The listing builds one solid part. Answer for the finished solid, in the listing's coordinates (mm). A direction names the side the tool comes from. Round coordinates to 2 decimals unless told otherwise and drop trailing zeros. Loops run counter-clockwise (first coordinate to the right, second up) from the corner with the lowest first, then second, coordinate; pieces in that order, holes last. Notation, with made-up numbers: (81, 74.25) -> (139, 74.25) arc R22 ccw to (139, 93.25) -> close; hole circle Ø1 at (64.25, 46.5). An arc over 180 degrees is marked (long way). One line per question, with ' | ' between items.
from build123d import *

# Parameters (mm, degrees)
SKETCH_1_W                   = 46
SKETCH_1_H                   = 26
EXTRUDE_1_DEPTH              = 3
SKETCH_2_W                   = 3
SKETCH_2_H                   = 26
EXTRUDE_2_DEPTH              = 34
CUT_EXTRUDE_START            = -46
CUT_EXTRUDE_1_DEPTH          = 46
SKETCH_4_R                   = 4
CUT_EXTRUDE_2_DEPTH          = 61.448325039
HOLE_START                   = -23
HOLE_WIZARD_M2_2_OUTLINE_R   = 2.2
HOLE_WIZARD_M2_2_DEPTH       = 2
HOLE_START_2                 = -21
HOLE_WIZARD_M2_2_2_OUTLINE_R = 1.2
HOLE_WIZARD_M2_2_2_DEPTH     = 1
CHAMFER_1_SIZE               = 3
SKETCH_15_W                  = 8
SKETCH_15_H                  = 5
CUT_EXTRUDE_8_DEPTH          = 11
CUT_EXTRUDE_9_DEPTH          = 44.058100283
CUT_EXTRUDE_9_DEPTH_BACK     = 44.058100283
SKETCH_18_W                  = 5
SKETCH_18_H                  = 5
HOLE_WIZARD_M2_4_D           = 2.4
HOLE_WIZARD_M2_4_CBORE_D     = 4.4
HOLE_WIZARD_M2_4_CBORE_DEPTH = 2


# Read off the part's stored shape, not the designer's step: 切除-拉伸1, M2 凹头盖螺钉的柱形沉头孔2
with BuildPart() as part:
    # 草图1 → 凸台-拉伸1 (new body)
    with BuildSketch(Plane(origin=(0, 0, 0), x_dir=(1, 0, 0), z_dir=(0, 1, 0))):
        Rectangle(SKETCH_1_W, SKETCH_1_H)
    extrude(amount=EXTRUDE_1_DEPTH)

    # 草图2 → 凸台-拉伸2 (add)
    with BuildSketch(Plane(origin=(0, 3, 0), x_dir=(1, 0, 0), z_dir=(0, 1, 0))):
        with Locations((-21.5, 0)):
            Rectangle(SKETCH_2_W, SKETCH_2_H)
        with Locations((21.5, 0)):
            Rectangle(SKETCH_2_W, SKETCH_2_H)
    extrude(amount=EXTRUDE_2_DEPTH)

    # 切除-拉伸1 outline → 切除-拉伸1 (cut)
    with BuildSketch(Plane.ZY.offset(23).offset(CUT_EXTRUDE_START)):
        with BuildLine():
            Line((13, 37), (0.412804961, 37))
            ThreePointArc((0.412804961, 37), (9.197021473, 33.197021473), (13, 24.412804961))
            Line((13, 24.412804961), (13, 37))
        make_face()
        with BuildLine():
            ThreePointArc((-13, 24.412804961), (-9.197021473, 33.197021473), (-0.412804961, 37))
            Line((-0.412804961, 37), (-13, 37))
            Line((-13, 37), (-13, 24.412804961))
        make_face()
    extrude(amount=CUT_EXTRUDE_1_DEPTH, mode=Mode.SUBTRACT)

    # 草图4 → 切除-拉伸2 (cut, through all)
    with BuildSketch(Plane.ZY.offset(23)):
        with Locations((0, 24.412804961)):
            Circle(SKETCH_4_R)
    extrude(amount=-CUT_EXTRUDE_2_DEPTH, mode=Mode.SUBTRACT)

    # M2 凹头盖螺钉的柱形沉头孔2 outline → M2 凹头盖螺钉的柱形沉头孔2 (cut)
    with BuildSketch(Plane.YZ.offset(HOLE_START)):
        with Locations((16.412804961, 0)):
            Circle(HOLE_WIZARD_M2_2_OUTLINE_R)
        with Locations((24.412804961, 8)):
            Circle(HOLE_WIZARD_M2_2_OUTLINE_R)
        with Locations((24.412804961, -8)):
            Circle(HOLE_WIZARD_M2_2_OUTLINE_R)
        with Locations((32.412804961, 0)):
            Circle(HOLE_WIZARD_M2_2_OUTLINE_R)
    hole_wizard_m2_2 = extrude(amount=HOLE_WIZARD_M2_2_DEPTH, mode=Mode.SUBTRACT)

    # Hole Wizard M2 _2 2 outline → Hole Wizard M2 _2 2 (cut)
    with BuildSketch(Plane.YZ.offset(HOLE_START_2)):
        with Locations((16.412804961, 0)):
            Circle(HOLE_WIZARD_M2_2_2_OUTLINE_R)
        with Locations((24.412804961, 8)):
            Circle(HOLE_WIZARD_M2_2_2_OUTLINE_R)
        with Locations((24.412804961, -8)):
            Circle(HOLE_WIZARD_M2_2_2_OUTLINE_R)
        with Locations((32.412804961, 0)):
            Circle(HOLE_WIZARD_M2_2_2_OUTLINE_R)
    hole_wizard_m2_2_2 = extrude(amount=HOLE_WIZARD_M2_2_2_DEPTH, mode=Mode.SUBTRACT)

    # 镜向2: M2 凹头盖螺钉的柱形沉头孔2, Hole Wizard M2 _2 2 across plane
    add(hole_wizard_m2_2.mirror(Plane(origin=(0, 0, 0), x_dir=(0, 0, 1), z_dir=(1, 0, 0))), mode=Mode.SUBTRACT)
    add(hole_wizard_m2_2_2.mirror(Plane(origin=(0, 0, 0), x_dir=(0, 0, 1), z_dir=(1, 0, 0))), mode=Mode.SUBTRACT)

    # 倒角1
    chamfer_1_edges = [part.edges().sort_by_distance(p)[0] for p in [
        (-23, 0, 0),
        (23, 0, 0),
    ]]
    chamfer(chamfer_1_edges, length=CHAMFER_1_SIZE)

    # 草图15 → 切除-拉伸8 (cut)
    with BuildSketch(Plane(origin=(23, 0, 0), x_dir=(0, 0, -1), z_dir=(1, 0, 0))):
        with Locations((0, 3.5)):
            Rectangle(SKETCH_15_W, SKETCH_15_H)
    cut_extrude_8 = extrude(amount=-CUT_EXTRUDE_8_DEPTH, mode=Mode.SUBTRACT)

    # 镜向3: 切除-拉伸8 across plane
    add(cut_extrude_8.mirror(Plane(origin=(0, 0, 0), x_dir=(0, 0, 1), z_dir=(1, 0, 0))), mode=Mode.SUBTRACT)

    # 草图18 → 切除-拉伸9 (cut, two sides: drawn at the far end of the back side and taken through both)
    with BuildSketch(Plane(origin=(0, 3, 0), x_dir=(1, 0, 0), z_dir=(0, 1, 0)).offset(-CUT_EXTRUDE_9_DEPTH_BACK)):
        Rectangle(SKETCH_18_W, SKETCH_18_H)
    extrude(amount=CUT_EXTRUDE_9_DEPTH + CUT_EXTRUDE_9_DEPTH_BACK, mode=Mode.SUBTRACT)

    # M2 凹头盖螺钉的柱形沉头孔4 (through all)
    with Locations(Plane(origin=(-5, 3, -5), x_dir=(0, 0, 1), z_dir=(0, 1, 0))):
        with Locations((0, 0), (5, 0), (10, 0), (10, 5), (10, 10), (5, 10), (0, 10), (0, 5)):
            CounterBoreHole(HOLE_WIZARD_M2_4_D / 2, HOLE_WIZARD_M2_4_CBORE_D / 2, HOLE_WIZARD_M2_4_CBORE_DEPTH)


solid = part.part
Q1. A cutting plane is placed at C-C on z = 8. Give the vertices of the cut face in (x, y), plus the area to 3 significant figures.
Numbers:
outline: (-23, 3) -> (-20, 0) -> (20, 0) -> (23, 3) -> (23, 22.21) -> (21, 22.21) -> (21, 23.21) -> (20, 23.21) -> (20, 3) -> (-20, 3) -> (-20, 23.21) -> (-21, 23.21) -> (-21, 22.21) -> (-23, 22.21) -> close; (-23, 26.61) -> (-21, 26.61) -> (-21, 25.61) -> (-20, 25.61) -> (-20, 34.26) -> (-23, 34.26) -> close; (20, 25.61) -> (21, 25.61) -> (21, 26.61) -> (23, 26.61) -> (23, 34.26) -> (20, 34.26) -> close | area: 294 mm^2
Q2. Given pin 1 Ø1.3 at (x, z) = (4.5, 4.5) entering from +Y; pin 2 Ø8 at (x, z) = (4.5, -3.5) entering from +Y; pin 3 Ø0.9 at (y, z) = (1, 0.5) entering from -X, each flat-ended and moving along its own axis, determine where each tip first touches the part or whether it passes through.
Numbers:
pin 1: y = 1 | pin 2: y = 3 | pin 3: x = -21
Q3. A cutting plane is placed at B-B on y = 4. Give the vertices of the cut face in (x, z).
Numbers:
outline: (-23, -13) -> (-20, -13) -> (-20, -4) -> (-23, -4) -> close; (-23, 4) -> (-20, 4) -> (-20, 13) -> (-23, 13) -> close; (20, -13) -> (23, -13) -> (23, -4) -> (20, -4) -> close; (20, 4) -> (23, 4) -> (23, 13) -> (20, 13) -> close
Q4. Find the intervals of material crossed by line 1 (X direction, y = 5.5, z = 11.25); line 2 (X direction, y = 24, z = -6); line 3 (Y direction, x = 1, z = -10), in increasing order. Write a range as from..to.
Numbers:
line 1: -23..-20, 20..23 | line 2: -21..-20, 20..21 | line 3: 0..3
Q5. A cutting plane is placed at A-A on x = 0. Give the vertices of the cut face in (y, z).
Numbers:
outline: (0, -13) -> (3, -13) -> (3, -7.2) -> (1, -7.2) -> (1, -6.2) -> (0, -6.2) -> close; (0, -3.8) -> (1, -3.8) -> (1, -2.8) -> (3, -2.8) -> (3, -2.5) -> (0, -2.5) -> close; (0, 2.5) -> (3, 2.5) -> (3, 2.8) -> (1, 2.8) -> (1, 3.8) -> (0, 3.8) -> close; (0, 6.2) -> (1, 6.2) -> (1, 7.2) -> (3, 7.2) -> (3, 13) -> (0, 13) -> close
Q6. For a pull along Z with two mould halves and no side action, classify faces 1 (the face through (-23, 20, 0)), 2 (the face through (6.19, 0.49, -4.84)) as pulls with the +Z half, pulls with the -Z half, needs draft (parallel to the pull), parting line crosses it, or undercut.
Numbers:
face 1: needs draft | face 2: undercut
Q7. A cutting plane is placed at D-D on y = 10. Give the vertices of the cut face in (x, z), plus the area to 3 significant figures.
Numbers:
outline: (-23, -13) -> (-20, -13) -> (-20, 13) -> (-23, 13) -> close; (20, -13) -> (23, -13) -> (23, 13) -> (20, 13) -> close | area: 156 mm^2
Q8. For faces 3 (the face through (4, 1, -4)), 4 (the face through (22.014, 34.445, -0.843)), 5 (the face through (-19, 2, 4)), 6 (the face through (-12, 2, 0)), 7 (the face through (22, 6, 0)), determine the directions among +Z, -Z, +X, -X, +Y, -Y from which every point of the face is accessible in a straight line to the end or side of a thin tool.
Numbers:
face 3: +Y | face 4: +X | face 5: -X | face 6: -X, +Y | face 7: +X, -X
